Verification items for the finished model (mm, model axes). A direction names the side the tool comes from. Give positions to 0.01 mm unless a question says otherwise; leave off trailing zeros. Loops run counter-clockwise (first coordinate to the right, second up) from the corner with the lowest first, then second, coordinate; pieces in that order, holes last. Notation, with made-up numbers: (-19.75, -9) - (38.25, -9) arc R20 cw to (38.25, 10) - close; hole circle Ø10 at (39, -30.5). An arc over 180 degrees is marked (long way). Answer in a Markdown table with one row per item.
```python
from build123d import *

# Parameters (mm, degrees)
SKETCH1_R           = 0.6477
BOSS_EXTRUDE1_DEPTH = 35.56
SKETCH3_R           = 0.6477
SKETCH4_R           = 0.6477
SKETCH4_R_2         = 0.381
CUT_EXTRUDE2_DEPTH  = 3.81


with BuildPart() as part:
    # Sketch1 → Boss-Extrude1 (new body)
    with BuildSketch(Plane.XY):
        Circle(SKETCH1_R)
    extrude(amount=BOSS_EXTRUDE1_DEPTH)

    # Sweep1: sweep along a path in Sketch2
    with BuildLine(Plane(origin=(0, 0, 0), x_dir=(1, 0, 0), z_dir=(0, 1, 0))) as sweep1_path:
        Line((3.4798, -50.8), (3.4798, -42.414004897))
        ThreePointArc((3.4798, -42.414004897), (3.286454013, -41.441988979), (2.735851224, -40.617953673))
        Line((2.735851224, -40.617953673), (0.743948776, -38.626051224))
        ThreePointArc((0.743948776, -38.626051224), (0.193345987, -37.802015918), (0, -36.83))
        Line((0, -36.83), (0, -35.56))
    # Sketch3 → Sweep1 (sweep)
    with BuildSketch(Plane.XY.offset(35.56)):
        Circle(SKETCH3_R)
    sweep(path=sweep1_path.line)

    # Sketch4 → Cut-Extrude2 (cut)
    with BuildSketch(Plane.XY):
        Circle(SKETCH4_R)
        Circle(SKETCH4_R_2, mode=Mode.SUBTRACT)
    extrude(amount=CUT_EXTRUDE2_DEPTH, mode=Mode.SUBTRACT)


solid = part.part
```
Q1. Sectioned sample at B-B (z = 18.5). Record the cut outline in (x, y).
Completed:
| item | result |
|---|---|
| outline | circle Ø1.3 at (0, 0) |
Q2. Tool access check on faces 1 (the face through (3, 0, 50.8)), 2 (the face through (2.833, -0.028, 46.548)), 3 (the face through (-0.14, 0.632, 20.089)). Record the directions out of +Z, -Z, +X, -X, +Y, -Y that give a thin tool (end or side, any length) a straight path to the whole face; none if there is none.
Completed:
| item | result |
|---|---|
| face 1 | +Z, +X, -X, +Y, -Y |
| face 2 | +Z |
| face 3 | -Z |
Q3. Thickness scan on line 1 (X direction, y = 0.1, z = 43); line 2 (Y direction, x = 0.1, z = 21). Record the ranges inside material, lowest first.
Completed:
| item | result |
|---|---|
| line 1 | 2.84 to 4.12 |
| line 2 | -0.64 to 0.64 |
Q4. Sectioned sample at A-A (y = 0). Record the cut outline in (x, z), and give its area (3 significant figures).
Completed:
| item | result |
|---|---|
| outline | (-0.65, 3.81) - (-0.38, 3.81) - (-0.38, 0) - (0.38, 0) - (0.38, 3.81) - (0.65, 3.81) - (0.65, 36.83) arc R1.89 cw to (1.2, 38.17) - (3.19, 40.16) arc R3.19 ccw to (4.13, 42.41) - (4.13, 50.8) - (2.83, 50.8) - (2.83, 42.41) arc R1.89 cw to (2.28, 41.08) - (0.29, 39.08) arc R3.19 ccw to (-0.65, 36.83) - close |
| area | 65.4 mm^2 |
